Geometry: final body of the model. Coordinates: model frame, mm. Coordinates: 2 decimals unless noted, no trailing zeros. Order: outer loops, then holes, each group sorted by start corner. A loop starts at its lowest first (then second) coordinate and runs counter-clockwise, first axis right, second up. Notation, with made-up numbers: M -35,64 L -16,64 A27 ccw -16,86 Z; hole C -39.5,7 d6. An arc over 180 degrees is marked long. Use CSV: the item, a comma, the result in double quotes. Start each with the question number.
1. Section query A-A on x = 100. Return the cut outline in (y, z) (3 decimals), and give its area (3 significant figures).
2. Section query B-B on y = -323.85. Return the cut outline in (x, z) (3 decimals), and give its area (3 significant figures).
3. Material intervals for line 1 (Y direction, x = 54.5, z = 41); line 2 (Y direction, x = 50, z = 37.5); line 3 (Z direction, x = 48, y = 323.85) (3 decimals), sorted ascending.
4. Section query C-C on z = -66. Return the cut outline in (x, y), and give its area (3 significant figures).
5. Pull-direction query (Y, two-part tool) for faces 1 (the cylindrical face through (81.394, -330.194, 41.554)), 2 (the flat face through (165.1, -5, 1)), 3 (the cylindrical face through (83.7, -318.7, -50.4)), 4 (the cylindrical face through (83.7, 318.7, -50.4)); classes: pulls with the +Y half, pulls with the -Y half, needs draft (parallel to the pull), parting line crosses it, or undercut.
6. First-contact query: P1, Ø12, axis at x = 122.5, z = -58.5, coming from the -Y side; P2, Ø1, axis at x = 79, z = 5.5, coming from the -Y side; P3, Ø1.5, axis at x = 110, z = -59, coming from the -Y side. Flat tips, straight axial feed; report the tip coordinate or a pass-through.
from build123d import *

# Parameters (mm, degrees)
F0_W     = 698.5
F0_H     = 158.75
F0_R     = 6.35
F1_DEPTH = 165.1
F2_R     = 101.6
F3_R     = 101.6


with BuildPart() as f1:
    # F0 (on Right) → F1 (new body)
    with BuildSketch(Plane.YZ):
        Rectangle(F0_W, F0_H)
        with Locations((-323.85, 41.275)):
            Circle(F0_R, mode=Mode.SUBTRACT)
        with Locations((323.85, 41.275)):
            Circle(F0_R, mode=Mode.SUBTRACT)
    extrude(amount=F1_DEPTH)

    # F2
    f2_edges = [f1.edges().sort_by_distance(p)[0] for p in [
        (82.55, 349.25, -79.375),
    ]]
    fillet(f2_edges, radius=F2_R)

    # F3
    f3_edges = [f1.edges().sort_by_distance(p)[0] for p in [
        (82.55, -349.25, -79.375),
    ]]
    fillet(f3_edges, radius=F3_R)


solid = f1.part
Results list:
1,outline,"M -349.25,22.225 A101.6 ccw -247.65,-79.375 L 247.65,-79.375 A101.6 ccw 349.25,22.225 L 349.25,79.375 L -349.25,79.375 Z; hole C -323.85,41.275 d12.7; hole C 323.85,41.275 d12.7"
1,area,"106,000 mm²"
2,outline,"M 0,-44.977 L 165.1,-44.977 L 165.1,34.925 L 0,34.925 Z; M 0,47.625 L 165.1,47.625 L 165.1,79.375 L 0,79.375 Z"
2,area,"18,400 mm²"
3,line 1,"y = -349.25 to -330.19, -317.51 to 317.51, 330.19 to 349.25"
3,line 2,"y = -349.25 to -328.96, -318.74 to 318.74, 328.96 to 349.25"
3,line 3,"z = -44.977 to 34.925, 47.625 to 79.375"
4,outline,"M 0,-298.04 L 165.1,-298.04 L 165.1,298.04 L 0,298.04 Z"
4,area,"98,400 mm²"
5,face 1,"undercut"
5,face 2,"needs draft"
5,face 3,"pulls with the -Y half"
5,face 4,"pulls with the +Y half"
6,P1,"stops at y = -316.49"
6,P2,"stops at y = -347.95"
6,P3,"stops at y = -309.67"
